Work out the finished part from the listing and answer in its coordinate system (mm). Give positions to 0.01 mm unless a question says otherwise; leave off trailing zeros. Loops run counter-clockwise (first coordinate to the right, second up) from the corner with the lowest first, then second, coordinate; pieces in that order, holes last. Notation, with made-up numbers: (69, 46.25) - (76, 46.25) arc R17 ccw to (76, 64.25) - close; hole circle Ø10 at (68.25, -2.75). An arc over 180 degrees is marked (long way). One line per item, written item: value.
from build123d import *


with BuildPart() as obj1:
    # Cone001 → Cone001 (revolve)
    with BuildSketch(Plane.XZ):
        Polygon((0, 0), (1.5, 0), (8, 10), (0, 10), align=None)
    revolve(axis=Axis((0, 0, 0), (0, 0, 1)))


with BuildPart() as obj2:
    # Cone → Cone (revolve)
    with BuildSketch(Plane.XZ):
        Polygon((0, 0), (3.5, 0), (10, 10), (0, 10), align=None)
    revolve(axis=Axis((0, 0, 0), (0, 0, 1)))

    # Cut: cut obj1
    add(obj1.part, mode=Mode.SUBTRACT)


solid = obj2.part
1. Flat-ended cylindrical pins translate along their axes: pin 1 Ø8 at (x, y) = (-2.5, -7.5) entering from -Z; pin 2 Ø3 at (x, z) = (-2, 1) entering from +Y; pin 3 Ø5 at (x, z) = (-7.5, 6) entering from -Y. Find the tip coordinate at first contact, or state that the pin passes through.
Output:
pin 1: stops at z = 0.62
pin 2: stops at y = 4.85
pin 3: stops at y = -6.34
2. Find the intervals of material crossed by line 1 along X through (y, z) = (-1.5, 5.25); line 2 along X through (y, z) = (2.25, 5.25); line 3 along Z through (x, y) = (5.75, 1.25), in increasing order.
Output:
line 1: x = -6.75 to -4.68, 4.68 to 6.75
line 2: x = -6.54 to -4.37, 4.37 to 6.54
line 3: z = 3.67 to 6.75
3. Section A-A (x = 0) is taken. Write down the section's boundary in (y, z).
Output:
outline: (-10, 10) - (-3.5, 0) - (-1.5, 0) - (-8, 10) - close; (1.5, 0) - (3.5, 0) - (10, 10) - (8, 10) - close
4. The mould has two halves that part along X. Classify faces 1 (the conical face through (4.415, 1.39, 1.737)), 2 (the conical face through (-2.66, -2.04, 2.85)), 3 (the flat face through (0, 8.2, 10)): released by +X, released by -X, zero draft, split by the parting line, or undercut.
Output:
face 1: split by the parting line
face 2: undercut
face 3: zero draft
5. Section C-C (z = 3) is taken. Write down the section's boundary in (x, y), and give its area (3 significant figures).
Output:
outline: circle Ø10.9 at (0, 0); hole circle Ø6.9 at (0, 0)
area: 55.9 mm²
6. Section D-D (z = 9.5) is taken. Write down the section's boundary in (x, y) (3 decimals), and give its area (3 significant figures).
Output:
outline: circle Ø19.35 at (0, 0); hole circle Ø15.35 at (0, 0)
area: 109 mm²
